Autodesk Inventor part; units mm, degrees
ref_plane "YZ Plane" through (0, 0, 0) normal (1, 0, 0) x (0, 1, 0)
ref_plane "XZ Plane" through (0, 0, 0) normal (0, 1, 0) x (-1, 0, 0)
ref_plane "XY Plane" through (0, 0, 0) normal (0, 0, 1) x (1, 0, 0)
sketch "Sketch1" plane through (0, 0, 0) normal (0, 1, 0) x (-1, 0, 0)
  line L0 (-7.5, 10) -> (7.5, 10)
  line L1 (7.5, 10) -> (7.5, -10)
  line L2 (7.5, -10) -> (-7.5, -10)
  line L3 (-7.5, -10) -> (-7.5, 10)
  line L4 (-7.5, 10) -> (7.5, -10) construction
  line L5 (7.5, 10) -> (-7.5, -10) construction
  point P0 (0, 0)
  dimension "d0" = 15
  dimension "d1" = 20
extrude "Extrusion1" add sketch "Sketch1" along normal mid plane 10
sketch "Sketch2" plane through (0, 5, 0) normal (0, 1, 0) x (1, 0, 0)
  line L0 (-3.5, 7) -> (-3.5, 10)
  line L1 (-3.5, 10) -> (-0.5, 10)
  line L2 (-0.5, 10) -> (-0.5, 9.3)
  line L3 (-0.5, 9.3) -> (-2.8, 9.3)
  line L4 (-2.8, 9.3) -> (-2.8, 7)
  line L5 (-2.8, 7) -> (-3.5, 7)
  line L6 (7.5, 10) -> (-7.5, 10)
  line L7 (-7.5, 10) -> (-7.5, -10)
  point P0 (0, 0)
  dimension "d4" = 3
  dimension "d5" = 0.7
  dimension "d7" = 4
extrude "Extrusion2" add sketch "Sketch2" along normal blind 1
fillet "Fillet1" radius 2 4 edges at (-7.5, 0, -10) (-7.5, 0, 10) (7.5, 0, 10) (7.5, 0, -10)
sketch "Sketch4" plane through (0, 5, 0) normal (0, 1, 0) x (1, 0, 0)
  line L0 (7.5, -8) -> (7.5, 8)
  line L1 (5.5, 10) -> (-0.5, 10)
  line L2 (-7.5, 8) -> (-7.5, -8)
  point P0 (0, 0)
  point P1 (5.5, 4)
  point P2 (-5.5, 4)
  dimension "d19" = 2
  dimension "d29" = 6
  dimension "d49" = 2
hole "Hole2" at (5.5, 5, -4) at (-5.5, 5, -4) direction (0, -1, 0) diameter 1.181 end through all
sketch "Sketch6" plane through (0, -5, 0) normal (0, -1, 0) x (1, 0, 0)
  line L0 (5.5, 10) -> (-5.5, 10)
  point P0 (0, 0)
  point P1 (0, 5)
  dimension "d38" = 5
hole "Hole4" at (0, -5, 5) direction (0, 1, 0) diameter 4.496 end through all
sketch "Sketch7" plane through (0, 5, 0) normal (0, 1, 0) x (1, 0, 0)
  circle A0 centre (0, -5) radius 2.248
  circle A1 centre (0, -5) radius 3.4
  point P0 (0, 0)
  dimension "d46" = 6.8
extrude "Extrusion3" cut sketch "Sketch7" against normal blind 4.3
properties part number "ChipHolder"
CAD build for the part. Positions are in the model's coordinates, mm. A direction names the side the tool comes from. Round coordinates to 2 decimals unless told otherwise and drop trailing zeros. Write each loop counter-clockwise with the first axis right and the second up, starting at its lowest first coordinate (ties: lowest second). Pieces come first, ordered by that corner, then holes.
Item 1: Band-saw the part on A-A on x = 0. Write the cut outline in (y, z), then the cut area to 3 significant figures.
Filled in:
outline: (-5, -10) - (5, -10) - (5, 1.6) - (0.7, 1.6) - (0.7, 2.75) - (-5, 2.75) - close; (-5, 7.25) - (0.7, 7.25) - (0.7, 8.4) - (5, 8.4) - (5, 10) - (-5, 10) - close
area: 145 mm2
Item 2: Band-saw the part on B-B on y = 0. Write the cut outline in (x, z).
Filled in:
outline: (-7.5, -8) arc R2 ccw to (-5.5, -10) - (5.5, -10) arc R2 ccw to (7.5, -8) - (7.5, 8) arc R2 ccw to (5.5, 10) - (-5.5, 10) arc R2 ccw to (-7.5, 8) - close; hole circle Ø1.18 at (-5.5, -4); hole circle Ø4.5 at (0, 5); hole circle Ø1.18 at (5.5, -4)
Item 3: Band-saw the part on D-D on z = 6.5. Write the cut outline in (x, y), then the cut area to 3 significant figures.
Filled in:
outline: (-7.5, -5) - (-1.67, -5) - (-1.67, 0.7) - (-3.05, 0.7) - (-3.05, 5) - (-7.5, 5) - close; (1.67, -5) - (7.5, -5) - (7.5, 5) - (3.05, 5) - (3.05, 0.7) - (1.67, 0.7) - close
area: 105 mm2
Item 4: Drop flat-ended pins along their axis: pin 1 Ø3 at (x, z) = (2, 7.5) entering from +Y; pin 2 Ø3.5 at (x, z) = (-1, 5) entering from +Y; pin 3 Ø0.5 at (y, z) = (5.5, -7.5) entering from +X. Give the stop position or say it passes through.
Filled in:
pin 1: stops at y = 5
pin 2: stops at y = 0.7
pin 3: stops at x = -2.8
Item 5: Band-saw the part on C-C on z = -4. Write the cut outline in (x, y).
Filled in:
outline: (-7.5, -5) - (-6.09, -5) - (-6.09, 5) - (-7.5, 5) - close; (-4.91, -5) - (4.91, -5) - (4.91, 5) - (-4.91, 5) - close; (6.09, -5) - (7.5, -5) - (7.5, 5) - (6.09, 5) - close
Item 6: Drill centre lines: L1, parallel to X at y = -0.25, z = -4; L2, parallel to Z at x = -5.5, y = 3; L3, parallel to X at y = -2, z = 5. Where is each one in solid material? Low to high.
Filled in:
L1: x = -7.5 to -6.09, -4.91 to 4.91, 6.09 to 7.5
L2: z = -10 to -4.59, -3.41 to 10
L3: x = -7.5 to -2.25, 2.25 to 7.5
Item 7: Tool access for faces 4 (the flat face through (-3.5, 5.5, -8.5)), 5 (the cylindrical face through (-0.44, 2.88, 1.63)), 6 (the flat face through (-1.6, 5.5, -9.3)): list every direction of +Z, -Z, +X, -X, +Y, -Y with a clear straight run to the whole face (end or side of a thin tool).
Filled in:
face 4: +Z, -Z, -X, +Y
face 5: +Y
face 6: +Z, +X, +Y
Item 8: Mould opens along X. For faces 1 (the cylindrical face through (-5.899, -0.07, -4.435)), 2 (the flat face through (0, -5, 0)), 3 (the flat face through (7.5, 0, 0)) say: released by +X, released by -X, zero draft, split by the parting line, or undercut.
Filled in:
face 1: undercut
face 2: zero draft
face 3: released by +X
